from build123d import *

# Parameters (mm, degrees)
SKETCH_1_W                   = 60
SKETCH_1_H                   = 60
EXTRUDE_1_DEPTH              = 5
SKETCH_3_W                   = 3
SKETCH_3_H                   = 3
EXTRUDE_3_DEPTH              = 10
CUT_EXTRUDE_1_DEPTH          = 67.136223055
CUT_EXTRUDE_2_DEPTH          = 10
PATTERN_CIRCULAR_1_COUNT     = 4
HOLE_WIZARD_M5_2_D           = 5.5
HOLE_WIZARD_M5_2_CBORE_D     = 11
HOLE_WIZARD_M5_2_CBORE_DEPTH = 3
EXTRUDE_4_DEPTH              = 10
CHAMFER_1_SIZE               = 1.5
SKETCH_10_W                  = 8
SKETCH_10_H                  = 8
EXTRUDE_5_DEPTH              = 10


with BuildPart() as part:
    # 스케치1 → 보스-돌출1 (new body)
    with BuildSketch(Plane.XY):
        Rectangle(SKETCH_1_W, SKETCH_1_H)
    extrude(amount=EXTRUDE_1_DEPTH)

    # 스케치3 → 보스-돌출3 (add)
    with BuildSketch(Plane.XY.offset(5)):
        with Locations((-28.5, -28.5)):
            Rectangle(SKETCH_3_W, SKETCH_3_H)
    extrude_3 = extrude(amount=EXTRUDE_3_DEPTH)

    # 스케치4 → 컷-돌출1 (cut, through all)
    with BuildSketch(Plane(origin=(-27, 0, 0), x_dir=(0, 0, -1), z_dir=(1, 0, 0))):
        Polygon((-15, -27), (-15, -28.5), (-5, -27), align=None)
    cut_extrude_1 = extrude(amount=-CUT_EXTRUDE_1_DEPTH, mode=Mode.SUBTRACT)

    # 스케치5 → 컷-돌출2 (cut)
    with BuildSketch(Plane.XZ.offset(30)):
        Polygon((-28.5, 15), (-27, 15), (-27, 5), align=None)
    cut_extrude_2 = extrude(amount=-CUT_EXTRUDE_2_DEPTH, mode=Mode.SUBTRACT)

    # 원형 패턴1: 보스-돌출3, 컷-돌출1, 컷-돌출2 ×4 about axis
    pattern_circular_1_axis = Axis((0, 0, 0), (0, 0, 1))
    add([extrude_3.rotate(pattern_circular_1_axis, i * 360 / PATTERN_CIRCULAR_1_COUNT) for i in range(1, PATTERN_CIRCULAR_1_COUNT)])
    add([cut_extrude_1.rotate(pattern_circular_1_axis, i * 360 / PATTERN_CIRCULAR_1_COUNT) for i in range(1, PATTERN_CIRCULAR_1_COUNT)], mode=Mode.SUBTRACT)
    add([cut_extrude_2.rotate(pattern_circular_1_axis, i * 360 / PATTERN_CIRCULAR_1_COUNT) for i in range(1, PATTERN_CIRCULAR_1_COUNT)], mode=Mode.SUBTRACT)

    # M5 소켓 머리 캡 나사용 카운터보어2 (through all)
    with Locations(Plane.XY.offset(5)):
        with Locations((-15, 15), (15, 15), (15, -15), (-15, -15)):
            CounterBoreHole(HOLE_WIZARD_M5_2_D / 2, HOLE_WIZARD_M5_2_CBORE_D / 2, HOLE_WIZARD_M5_2_CBORE_DEPTH)

    # 스케치9 → 보스-돌출4 (add)
    with BuildSketch(Plane(origin=(0, 0, 0), x_dir=(-1, 0, 0), z_dir=(0, 0, -1))):
        with BuildLine():
            Line((-20.05, 2.5), (-20.05, 8.545042831))
            ThreePointArc((-20.05, 8.545042831), (-15, 10.5), (-9.95, 8.545042831))
            Line((-9.95, 8.545042831), (-9.95, 2.5))
            Line((-9.95, 2.5), (-11.95, 2.5))
            Line((-11.95, 2.5), (-11.95, -2.5))
            Line((-11.95, -2.5), (-9.95, -2.5))
            Line((-9.95, -2.5), (-9.95, -8.545042831))
            ThreePointArc((-9.95, -8.545042831), (-15, -10.5), (-20.05, -8.545042831))
            Line((-20.05, -8.545042831), (-20.05, -2.5))
            Line((-20.05, -2.5), (-18.05, -2.5))
            Line((-18.05, -2.5), (-18.05, 2.5))
            Line((-18.05, 2.5), (-20.05, 2.5))
        make_face()
        with BuildLine():
            Line((2.5, 20.05), (8.545042831, 20.05))
            ThreePointArc((8.545042831, 20.05), (10.5, 15), (8.545042831, 9.95))
            Line((8.545042831, 9.95), (2.5, 9.95))
            Line((2.5, 9.95), (2.5, 11.95))
            Line((2.5, 11.95), (-2.5, 11.95))
            Line((-2.5, 11.95), (-2.5, 9.95))
            Line((-2.5, 9.95), (-8.545042831, 9.95))
            ThreePointArc((-8.545042831, 9.95), (-10.5, 15), (-8.545042831, 20.05))
            Line((-8.545042831, 20.05), (-2.5, 20.05))
            Line((-2.5, 20.05), (-2.5, 18.05))
            Line((-2.5, 18.05), (2.5, 18.05))
            Line((2.5, 18.05), (2.5, 20.05))
        make_face()
        with BuildLine():
            Line((20.05, -2.5), (20.05, -8.545042831))
            ThreePointArc((20.05, -8.545042831), (15, -10.5), (9.95, -8.545042831))
            Line((9.95, -8.545042831), (9.95, -2.5))
            Line((9.95, -2.5), (11.95, -2.5))
            Line((11.95, -2.5), (11.95, 2.5))
            Line((11.95, 2.5), (9.95, 2.5))
            Line((9.95, 2.5), (9.95, 8.545042831))
            ThreePointArc((9.95, 8.545042831), (15, 10.5), (20.05, 8.545042831))
            Line((20.05, 8.545042831), (20.05, 2.5))
            Line((20.05, 2.5), (18.05, 2.5))
            Line((18.05, 2.5), (18.05, -2.5))
            Line((18.05, -2.5), (20.05, -2.5))
        make_face()
        with BuildLine():
            Line((-2.5, -20.05), (-8.545042831, -20.05))
            ThreePointArc((-8.545042831, -20.05), (-10.5, -15), (-8.545042831, -9.95))
            Line((-8.545042831, -9.95), (-2.5, -9.95))
            Line((-2.5, -9.95), (-2.5, -11.95))
            Line((-2.5, -11.95), (2.5, -11.95))
            Line((2.5, -11.95), (2.5, -9.95))
            Line((2.5, -9.95), (8.545042831, -9.95))
            ThreePointArc((8.545042831, -9.95), (10.5, -15), (8.545042831, -20.05))
            Line((8.545042831, -20.05), (2.5, -20.05))
            Line((2.5, -20.05), (2.5, -18.05))
            Line((2.5, -18.05), (-2.5, -18.05))
            Line((-2.5, -18.05), (-2.5, -20.05))
        make_face()
    extrude(amount=EXTRUDE_4_DEPTH)

    # 모따기1
    chamfer_1_edges = [part.edges().sort_by_distance(p)[0] for p in [
        (15, -10.5, -10),
        (9.95, -5.522521416, -10),
        (10.95, -2.5, -10),
        (11.95, 0, -10),
        (10.95, 2.5, -10),
        (9.95, 5.522521416, -10),
        (15, 10.5, -10),
        (20.05, 5.522521416, -10),
        (19.05, 2.5, -10),
        (18.05, 0, -10),
        (19.05, -2.5, -10),
        (20.05, -5.522521416, -10),
        (10.5, 15, -10),
        (5.522521416, 9.95, -10),
        (2.5, 10.95, -10),
        (0, 11.95, -10),
        (-2.5, 10.95, -10),
        (-5.522521416, 9.95, -10),
        (-10.5, 15, -10),
        (-5.522521416, 20.05, -10),
        (-2.5, 19.05, -10),
        (0, 18.05, -10),
        (2.5, 19.05, -10),
        (5.522521416, 20.05, -10),
        (-15, 10.5, -10),
        (-9.95, 5.522521416, -10),
        (-10.95, 2.5, -10),
        (-11.95, 0, -10),
        (-10.95, -2.5, -10),
        (-9.95, -5.522521416, -10),
        (-15, -10.5, -10),
        (-20.05, -5.522521416, -10),
        (-19.05, -2.5, -10),
        (-18.05, 0, -10),
        (-19.05, 2.5, -10),
        (-20.05, 5.522521416, -10),
        (-10.5, -15, -10),
        (-5.522521416, -9.95, -10),
        (-2.5, -10.95, -10),
        (0, -11.95, -10),
        (2.5, -10.95, -10),
        (5.522521416, -9.95, -10),
        (10.5, -15, -10),
        (5.522521416, -20.05, -10),
        (2.5, -19.05, -10),
        (0, -18.05, -10),
        (-2.5, -19.05, -10),
        (-5.522521416, -20.05, -10),
    ]]
    chamfer(chamfer_1_edges, length=CHAMFER_1_SIZE)

    # 스케치10 → 보스-돌출5 (add)
    with BuildSketch(Plane.XY.offset(5)):
        Rectangle(SKETCH_10_W, SKETCH_10_H)
    extrude(amount=EXTRUDE_5_DEPTH)


solid = part.part
Can you work these out from the model? Positions are in its coordinate system, mm. A direction names the side the tool comes from. Coordinates: 2 decimals unless noted, no trailing zeros. Order: outer loops, then holes, each group sorted by start corner. A loop starts at its lowest first (then second) coordinate and runs counter-clockwise, first axis right, second up. Notation, with made-up numbers: (31, 5.25) - (44, 5.25) arc R24 cw to (44, 21.25) - close; hole circle Ø8 at (14.5, 5.25). An arc over 180 degrees is marked (long way). Answer as a JSON object with one key per item and string values. Group by question number.
Q1. Imagine slicing it at D-D (x = -6.5). Please give me the cut outline in (y, z), and give its area (4 significant figures).
Q2. I need wall thicknesses on line 1 (Y direction, x = -15, z = 4.2); line 2 (Y direction, x = 15, z = 1.15); line 3 (Y direction, x = -4.5, z = -8.25). Which ranges of each line are inside material? Lowest first, please. Write a range as from..to.
Q3. Will these pins go through, and if not, where does the flat tip stop? P1, Ø2.5, axis at x = -2, z = 12.5, coming from the -Y side; P2, Ø3, axis at y = 6, z = -4.5, coming from the -X side; P3, Ø1.8, axis at y = -4.5, z = -4.5, coming from the +X side.
Q4. We'd pull the mould along X, two halves only. Please class faces 1 (the face through (11, -2.5, -4)), 2 (the face through (-18, -16, 2)), 3 (the face through (5.56, 19.29, -9.26)): +X half, -X half, draft (parallel to the pull), parting line (faces both ways), or undercut.
Q5. Imagine slicing it at A-A (x = -15). Please give me the cut outline in (y, z), and give its area (3 significant figures).
Q6. Imagine slicing it at C-C (z = 11). Please give me the cut outline in (x, y).
Q7. On a 3-axis mill with a long thin cutter (end or side, diameter ignored), from which of +Z, -Z, +X, -X, +Y, -Y can I reach the whole of each face in a straight line? I mean faces 4 (the face through (12, -16, 2)), 5 (the face through (-18, -3, -9)), 6 (the face through (19, 2.5, -4)), 7 (the face through (-11, 2.5, -4)). Say none if no direction works.
Determined:
{
 "1": {"outline": "(-30, 0) - (-20.05, 0) - (-20.05, -8.5) - (-18.55, -10) - (-11.45, -10) - (-9.95, -8.5) - (-9.95, 0) - (9.95, 0) - (9.95, -8.5) - (11.45, -10) - (18.55, -10) - (20.05, -8.5) - (20.05, 0) - (30, 0) - (30, 5) - (-30, 5) - close", "area": "497.5 mm2"},
 "2": {"line 1": "y = -30..-20.5, -9.5..9.5, 20.5..30", "line 2": "y = -30..-17.75, -12.25..12.25, 17.75..30", "line 3": "y = -20.05..-9.95, 9.95..20.05"},
 "3": {"P1": "stops at y = -4", "P2": "stops at x = -20.05", "P3": "stops at x = 20.05"},
 "4": {"face 1": "undercut", "face 2": "undercut", "face 3": "draft"},
 "5": {"outline": "(-30, 0) - (-17.75, 0) - (-17.75, 2) - (-20.5, 2) - (-20.5, 5) - (-30, 5) - close; (-12.25, 0) - (-10.5, 0) - (-10.5, -8.5) - (-9, -10) - (9, -10) - (10.5, -8.5) - (10.5, 0) - (12.25, 0) - (12.25, 2) - (9.5, 2) - (9.5, 5) - (-9.5, 5) - (-9.5, 2) - (-12.25, 2) - close; (17.75, 0) - (30, 0) - (30, 5) - (20.5, 5) - (20.5, 2) - (17.75, 2) - close", "area": "420 mm2"},
 "6": {"outline": "(-30, -30) - (-27.9, -30) - (-27.9, -27.9) - (-30, -27.9) - close; (-30, 27.9) - (-27.9, 27.9) - (-27.9, 30) - (-30, 30) - close; (-4, -4) - (4, -4) - (4, 4) - (-4, 4) - close; (27.9, -30) - (30, -30) - (30, -27.9) - (27.9, -27.9) - close; (27.9, 27.9) - (30, 27.9) - (30, 30) - (27.9, 30) - close"},
 "7": {"face 4": "+Z", "face 5": "-Z, -X", "face 6": "-Z, +X", "face 7": "-Z"}
}
